Part model, mm, in its own coordinate system. A direction names the side the tool comes from. Round coordinates to 2 decimals unless told otherwise and drop trailing zeros. Loops run counter-clockwise (first coordinate to the right, second up) from the corner with the lowest first, then second, coordinate; pieces in that order, holes last.
(1) Cut at B-B on y = 12.5. List the corners of the cut face in (x, z).
(2) Tool access for faces 1 (the face through (20.301, 9.114, 2.87)), 2 (the face through (2.46, -1.86, 14.13)): list every direction of +Z, -Z, +X, -X, +Y, -Y with a clear straight run to the whole face (end or side of a thin tool).
(3) Cut at A-A on x = 9.5. List the corners of the cut face in (y, z), then the cut area to 3 significant figures.
(4) Flat gauge pins, fed straight in: pin 1 (3 mm diameter, centred on x = 26.5, y = -6.5, fed in from -Z); pin 2 (4 mm diameter, centred on x = 6, y = 3.5, fed in from -Z); pin 3 (2 mm diameter, centred on x = 4.5, y = 8.5, fed in from -Z). Where does each tip first touch, or does it go through?
(5) Probe probe 1 along Z at (x, y) = (26.5, 0.25); probe 2 along X at (y, z) = (7.25, -12); probe 3 along X at (y, z) = (-5.5, 4). List the from-to ranges inside material, lowest first.
(6) Cut at C-C on x = 3. List the corners of the cut face in (y, z), then the cut area to 3 significant figures.
from build123d import *

# Parameters (mm, degrees)
F0_R      = 5.258166692
F12_DEPTH = 45
F1_R      = 9.5550685652
F2_DEPTH  = 39
F13_R     = 14.2505021401
F3_DEPTH  = 5
F4_R      = 2
F6_R      = 2
F10_W     = 1.8654689193
F10_H     = 2.0018368959
F11_DEPTH = 45


# Not quite as in the source:
# - a fillet or chamfer that OpenCascade refuses, or shapes differently, is made with other operations: its cross-section is extruded or revolved along the edge and cut away or added
# - the program builds the solid bodies; features that only make, move or delete a surface that nothing else refers to are left out


with BuildPart() as f12:
    # F0 (on Right) → F12 (new body)
    with BuildSketch(Plane.YZ):
        Circle(F0_R)
    extrude(amount=F12_DEPTH)

    # F1 (on Right) → F2 (join)
    with BuildSketch(Plane.YZ):
        Circle(F1_R)
    extrude(amount=F2_DEPTH)

    # F13 (on Right) → F3 (join)
    with BuildSketch(Plane.YZ):
        Circle(F13_R)
    extrude(amount=F3_DEPTH)

    # F4
    f4_edges = [f12.edges().sort_by_distance(p)[0] for p in [
        (45, -5.258167, 0),
    ]]
    fillet(f4_edges, radius=F4_R)

    # F5: fillet of radius 5.08 on 1 edges, made by hand

    # F5_s1 → F5_t2 (revolve, cut)
    with BuildSketch(Plane.XY):
        with BuildLine():
            ThreePointArc((39, 5.258166692), (37.2843755862, 8.3341188683), (33.9807214339, 9.5550685652))
            Line((33.9807214339, 9.5550685652), (39, 9.5550685652))
            Line((39, 9.5550685652), (39, 5.258166692))
        make_face()
    revolve(axis=Axis((39, 0, 0), (1, 0, 0)), mode=Mode.SUBTRACT)

    # F6
    f6_edges = [f12.edges().sort_by_distance(p)[0] for p in [
        (5, -9.555069, 0),
    ]]
    fillet(f6_edges, radius=F6_R)

    # F10 (on Right) → F11 (join)
    with BuildSketch(Plane.YZ):
        Rectangle(F10_W, F10_H)
    extrude(amount=F11_DEPTH)


solid = f12.part
Final values:
1. outline: (0, -6.84) - (5, -6.84) - (5, 6.84) - (0, 6.84) - close
2. face 1: +X
2. face 2: +X, -X
3. outline: circle Ø19.11 at (0, 0)
3. area: 287 mm2
4. pin 1: stops at z = -8.14
4. pin 2: stops at z = -14.14
4. pin 3: stops at z = -12.12
5. probe 1: z = -9.55 to 9.55
5. probe 2: x = 0 to 5
5. probe 3: x = 0 to 38.5
6. outline: circle Ø28.5 at (0, 0)
6. area: 638 mm2
